Geometry: final body of the model. Coordinates: model frame, mm. A direction names the side the tool comes from. Round coordinates to 2 decimals unless told otherwise and drop trailing zeros. Write each loop counter-clockwise with the first axis right and the second up, starting at its lowest first coordinate (ties: lowest second). Pieces come first, ordered by that corner, then holes. Notation, with made-up numbers: M 48,22.25 L 102,22.25 A18 cw 102,31.25 Z; hole C 61.5,40 d5. An arc over 180 degrees is marked long. Use one line per item in the form item = value. Start each with the question number.
Autodesk Inventor part; units mm, degrees
ref_plane "YZ Plane" through (0, 0, 0) normal (1, 0, 0) x (0, 1, 0)
ref_plane "XZ Plane" through (0, 0, 0) normal (0, 1, 0) x (-1, 0, 0)
ref_plane "XY Plane" through (0, 0, 0) normal (0, 0, 1) x (1, 0, 0)
sketch "Sketch1" plane through (0, 0, 0) normal (0, 0, 1) x (1, 0, 0)
  circle A0 centre (0, 0) radius 3.5
  circle A1 centre (0, 0) radius 10.75
  dimension "d0" = 7
  dimension "d1" = 21.5
extrude "Extrusion1" add sketch "Sketch1" along normal blind 5.1
sketch "Sketch2" plane through (0, 0, 5.1) normal (0, 0, 1) x (1, 0, 0)
  circle A0 centre (0, 0) radius 10.75
  circle A1 centre (0, 0) radius 3.5
  circle A2 centre (0, 0) radius 5.5
  circle A3 centre (0, 0) radius 9.25
  dimension "d4" = 11
  dimension "d5" = 18.5
sketch "Sketch3" plane through (0, 0, 0) normal (0, 0, -1) x (-1, 0, 0)
  circle A0 centre (0, 0) radius 9.25
  circle A1 centre (0, 0) radius 5.5
  circle A2 centre (0, 0) radius 3.5
  circle A3 centre (0, 0) radius 10.75
extrude "Extrusion2" add sketch "Sketch3" along normal blind 1
extrude "Extrusion3" add sketch "Sketch2" along normal blind 1
properties part number "Cojinete"
1. Contact query for flat-ended pins moving along their axis: pin 1 (8 mm diameter, centred on x = 0, y = 0, fed in from +Z); pin 2 (3 mm diameter, centred on x = -3, z = 2.5, fed in from -Y); pin 3 (1 mm diameter, centred on x = 8.5, z = 0, fed in from -Y); pin 4 (4 mm diameter, centred on x = 0, y = 0, fed in from -Z). Output: stop coordinate, or through.
2. Set-up query: faces 3 (the face through (-4, 0, -1)), 4 (the face through (-2.01, 9.03, 5.59)), 5 (the face through (4, -4, 0)). Return all of +Z, -Z, +X, -X, +Y, -Y with unobstructed straight access to the full face (end or side cutting, diameter ignored); none if empty.
3. Pull-direction query (Y, two-part tool) for faces 1 (the face through (-5, 8, -1)), 2 (the face through (1.19, 5.37, -0.49)); classes: released by +Y, released by -Y, zero draft, split by the parting line, or undercut.
4. Section query A-A (x = 0). Return loops of the section in (y, z), then the cut area to 4 significant figures.
5. Section query C-C (y = -6.5). Return loops of the section in (x, z).
6. Ray query, probe 1 along Y at (x, z) = (0, -0.5); probe 2 along X at (y, z) = (0, 3); probe 3 along Z at (x, y) = (5, -4). Return the intervals inside material, ascending.
7. Section query D-D (x = 4.5). Return loops of the section in (y, z).
Checks:
q1.pin_1 = 6.1
q1.pin_2 = -10.64
q1.pin_3 = -7.18
q1.pin_4 = through
q2.face_3 = -Z, +X, -X, +Y, -Y
q2.face_4 = +Z
q2.face_5 = -Z
q3.face_1 = zero draft
q3.face_2 = undercut
q4.outline = M -10.75,-1 L -9.25,-1 L -9.25,0 L -5.5,0 L -5.5,-1 L -3.5,-1 L -3.5,6.1 L -5.5,6.1 L -5.5,5.1 L -9.25,5.1 L -9.25,6.1 L -10.75,6.1 Z; M 3.5,-1 L 5.5,-1 L 5.5,0 L 9.25,0 L 9.25,-1 L 10.75,-1 L 10.75,6.1 L 9.25,6.1 L 9.25,5.1 L 5.5,5.1 L 5.5,6.1 L 3.5,6.1 Z
q4.area = 87.95 mm^2
q5.outline = M -8.56,-1 L -6.58,-1 L -6.58,0 L 6.58,0 L 6.58,-1 L 8.56,-1 L 8.56,6.1 L 6.58,6.1 L 6.58,5.1 L -6.58,5.1 L -6.58,6.1 L -8.56,6.1 Z
q6.probe_1 = -10.75 to -9.25, -5.5 to -3.5, 3.5 to 5.5, 9.25 to 10.75
q6.probe_2 = -10.75 to -3.5, 3.5 to 10.75
q6.probe_3 = 0 to 5.1
q7.outline = M -9.76,-1 L -8.08,-1 L -8.08,0 L -3.16,0 L -3.16,-1 L 3.16,-1 L 3.16,0 L 8.08,0 L 8.08,-1 L 9.76,-1 L 9.76,6.1 L 8.08,6.1 L 8.08,5.1 L 3.16,5.1 L 3.16,6.1 L -3.16,6.1 L -3.16,5.1 L -8.08,5.1 L -8.08,6.1 L -9.76,6.1 Z
